Model file for the job. Use its own axes, mm. A direction names the side the tool comes from. Give positions to 0.01 mm unless a question says otherwise; leave off trailing zeros. Loops run counter-clockwise (first coordinate to the right, second up) from the corner with the lowest first, then second, coordinate; pieces in that order, holes last. Notation, with made-up numbers: M 0,22 L 55,22 A21 ccw 55,45 Z; hole C 24,11 d11. An arc over 180 degrees is marked long. Answer in a Markdown table with one row per item.
```python
from build123d import *

# Parameters (mm, degrees)
SKETCH1_W                = 8
SKETCH1_H                = 10
BOSS_EXTRUDE1_DEPTH      = 2
SKETCH2_W                = 6.2
SKETCH2_H                = 10
CUT_EXTRUDE1_DEPTH       = 1
BOSS_EXTRUDE2_DEPTH      = 1.5
BOSS_EXTRUDE2_DEPTH_BACK = 1
M1_CLEARANCE_HOLE2_D     = 1.2
M1_CLEARANCE_HOLE2_DEPTH = 5
M1_CLEARANCE_HOLE2_TIP   = 0.360516371
M1_CLEARANCE_HOLE1_D     = 1
M1_CLEARANCE_HOLE1_DEPTH = 5
M1_CLEARANCE_HOLE1_TIP   = 0.30043031
SKETCH8_R                = 0.4
CUT_EXTRUDE2_DEPTH       = 1.5
FILLET2_R                = 1


with BuildPart() as part:
    # Sketch1 → Boss-Extrude1 (new body)
    with BuildSketch(Plane.XY):
        with Locations((4, -5)):
            Rectangle(SKETCH1_W, SKETCH1_H)
    extrude(amount=BOSS_EXTRUDE1_DEPTH)

    # Sketch2 → Cut-Extrude1 (cut)
    with BuildSketch(Plane.XY.offset(2)):
        with Locations((4, -5)):
            Rectangle(SKETCH2_W, SKETCH2_H)
    extrude(amount=-CUT_EXTRUDE1_DEPTH, mode=Mode.SUBTRACT)

    # Sketch3 → Boss-Extrude2 (add, two sides)
    with BuildSketch(Plane(origin=(0, 0, 0), x_dir=(-1, 0, 0), z_dir=(0, 0, -1))) as boss_extrude2_sk:
        Polygon((-8, -10), (-4, -0.343145751), (0, -10), (-2.309698831, -10.956708581), (-4, -6.875960575), (-5.690301169, -10.956708581), align=None)
    extrude(amount=BOSS_EXTRUDE2_DEPTH)
    extrude(boss_extrude2_sk.sketch, amount=-BOSS_EXTRUDE2_DEPTH_BACK)

    # M1 Clearance Hole2
    with Locations(Plane(origin=(-3.535533906, -8.535533906, 0), x_dir=(-0.923879533, 0.382683432, 0), z_dir=(-0.382683432, -0.923879533, 0))):
        with Locations((-5.115994416, 0.25)):
            Hole(M1_CLEARANCE_HOLE2_D / 2, depth=M1_CLEARANCE_HOLE2_DEPTH)
            with Locations((0, 0, -(M1_CLEARANCE_HOLE2_DEPTH + M1_CLEARANCE_HOLE2_TIP / 2))):  # 118° drill point
                Cone(0, M1_CLEARANCE_HOLE2_D / 2, M1_CLEARANCE_HOLE2_TIP, mode=Mode.SUBTRACT)

    # M1 Clearance Hole1
    with Locations(Plane(origin=(4.707106781, -11.363961031, 0), x_dir=(-0.923879533, -0.382683432, 0), z_dir=(0.382683432, -0.923879533, 0))):
        with Locations((-2.314201936, 0.25)):
            Hole(M1_CLEARANCE_HOLE1_D / 2, depth=M1_CLEARANCE_HOLE1_DEPTH)
            with Locations((0, 0, -(M1_CLEARANCE_HOLE1_DEPTH + M1_CLEARANCE_HOLE1_TIP / 2))):  # 118° drill point
                Cone(0, M1_CLEARANCE_HOLE1_D / 2, M1_CLEARANCE_HOLE1_TIP, mode=Mode.SUBTRACT)

    # Sketch8 → Cut-Extrude2 (cut)
    with BuildSketch(Plane(origin=(0, 0, -1.5), x_dir=(-1, 0, 0), z_dir=(0, 0, -1))):
        with Locations((-4, -7.3)):
            Circle(SKETCH8_R)
    extrude(amount=-CUT_EXTRUDE2_DEPTH, mode=Mode.SUBTRACT)

    # Fillet2
    fillet2_edges = [part.edges().sort_by_distance(p)[0] for p in [
        (2.705980501, -10, 0.5),
        (5.294019499, -10, 0.5),
    ]]
    fillet(fillet2_edges, radius=FILLET2_R)


solid = part.part
```
Q1. Saw through at B-B (z = 0.85). Give the cut face in (x, y).
Reported:
| item | result |
|---|---|
| outline | M 0,-10 L 2.31,-10.96 L 2.45,-10.62 A1 cw 3.37,-10 L 4.63,-10 A1 cw 5.55,-10.62 L 5.69,-10.96 L 8,-10 L 8,0 L 0,0 Z |
Q2. Mould opens along Z. For faces 6 (the face through (4, -10, 0.5)), 7 (the face through (4.896, -5.605, -0.309)), 8 (the face through (4, -9, 0)), 9 (the face through (7.5, -4.9, 2)) say: released by +Z, released by -Z, zero draft, split by the parting line, or undercut.
Reported:
| item | result |
|---|---|
| face 6 | zero draft |
| face 7 | undercut |
| face 8 | released by -Z |
| face 9 | released by +Z |
Q3. Saw through at C-C (x = 7.5). Give the cut face in (y, z), and give its area (3 significant figures).
Reported:
| item | result |
|---|---|
| outline | M -10.21,-1.5 L -8.79,-1.5 L -8.79,0 L 0,0 L 0,2 L -10,2 L -10,1 L -10.21,1 Z |
| area | 22.3 mm² |
Q4. Drop flat-ended pins along their axis: pin 1 (1 mm diameter, centred on y = -3, z = -1, fed in from +X); pin 2 (0.5 mm diameter, centred on y = -7.5, z = 1.5, fed in from -X); pin 3 (1 mm diameter, centred on x = 4, y = -8.5, fed in from +Z); pin 4 (0.5 mm diameter, centred on x = 4, z = 0.5, fed in from -Y). Give the stop position or say it passes through.
Reported:
| item | result |
|---|---|
| pin 1 | x = 5.31 |
| pin 2 | x = 0 |
| pin 3 | z = 1 |
| pin 4 | y = -10 |
Q5. Probe probe 1 along X at (y, z) = (-0.5, 1.85); probe 2 along X at (y, z) = (-9.25, 0.05); probe 3 along Z at (x, y) = (3.75, -8.5). List the from-to ranges inside material, lowest first.
Reported:
| item | result |
|---|---|
| probe 1 | 0 to 0.9, 7.1 to 8 |
| probe 2 | 0 to 1.14, 2.27 to 5.9, 6.77 to 8 |
| probe 3 | 0 to 1 |
Q6. Saw through at A-A (z = 1.7). Give the cut face in (x, y), and give its area (3 significant figures).
Reported:
| item | result |
|---|---|
| outline | M 0,-10 L 0.9,-10 L 0.9,0 L 0,0 Z; M 7.1,-10 L 8,-10 L 8,0 L 7.1,0 Z |
| area | 18.0 mm² |
Q7. Saw through at D-D (y = -7.25). Give the number of separate pieces and of enclosed holes in the cut face, and give its area (3 significant figures).
Reported:
| item | result |
|---|---|
| separate pieces | 1 |
| enclosed holes | 2 |
| area | 15.1 mm² |
Q8. 3-axis set-ups, long thin cutter, end or side, ignore diameter. For faces 1 (the face through (5.188, -10.173, 0.493)), 2 (the face through (3.13, -5.56, -0.21)), 3 (the face through (2.03, -5.1, -0.74)), 4 (the face through (7.5, -10, 1.5)), 5 (the face through (4.98, -9.24, -0.82)): which of +Z, -Z, +X, -X, +Y, -Y reach the whole face in a straight line?
Reported:
| item | result |
|---|---|
| face 1 | +Z, -Z, -Y |
| face 2 | none |
| face 3 | -Z, -X, +Y |
| face 4 | +Z, +X, -X, -Y |
| face 5 | -Z, -Y |
